Design review of the part built by this model. Coordinates are the model's own, in mm. Give positions to 0.01 mm unless a question says otherwise; leave off trailing zeros. Write each loop counter-clockwise with the first axis right and the second up, starting at its lowest first coordinate (ties: lowest second). Pieces come first, ordered by that corner, then holes. Notation, with made-up numbers: M -5.5,37 L 8.5,37 A18 ccw 8.5,58 Z; hole C 56,65 d5. An arc over 180 degrees is marked long. Use one line per item in the form item = value. Start each with the question number.
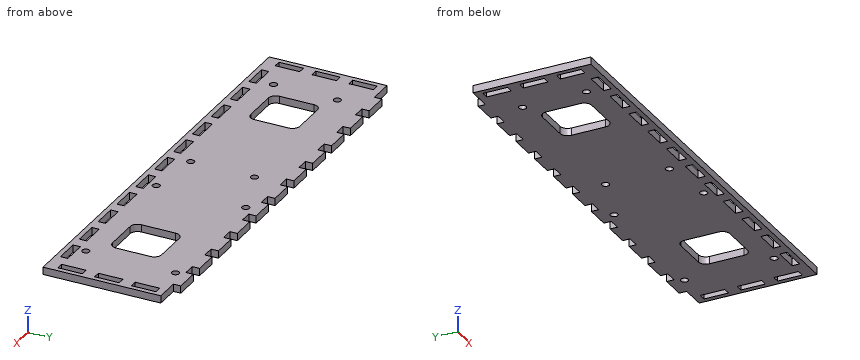
from build123d import *

# Parameters (mm, degrees)
SKETCH_1_W          = 3
SKETCH_1_H          = 10
SKETCH_1_W_2        = 10
SKETCH_1_H_2        = 3
EXTRUDE_1_DEPTH     = 3
SKETCH_2_W          = 20
SKETCH_2_H          = 20
CUT_EXTRUDE_1_DEPTH = 10
FILLET_1_R          = 3
SKETCH_3_R          = 1.5
CUT_EXTRUDE_2_DEPTH = 10


with BuildPart() as part:
    # 草图1 → 凸台-拉伸1 (new body)
    with BuildSketch(Plane.XY):
        Polygon((-90, 24), (-80, 24), (-80, 27), (-70, 27), (-70, 24), (-65, 24), (-65, 27), (-55, 27), (-55, 24), (-50, 24), (-50, 27), (-40, 27), (-40, 24), (-35, 24), (-35, 27), (-25, 27), (-25, 24), (-20, 24), (-20, 27), (-10, 27), (-10, 24), (-5, 24), (-5, 27), (5, 27), (5, 24), (10, 24), (10, 27), (20, 27), (20, 24), (25, 24), (25, 27), (35, 27), (35, 24), (40, 24), (40, 27), (50, 27), (50, 24), (55, 24), (55, 27), (65, 27), (65, 24), (70, 24), (70, 27), (80, 27), (80, 24), (90, 24), (90, -24), (-90, -24), align=None)
        with Locations((-86.5, 1)):
            Rectangle(SKETCH_1_W, SKETCH_1_H, mode=Mode.SUBTRACT)
        with Locations((-86.5, 16)):
            Rectangle(SKETCH_1_W, SKETCH_1_H, mode=Mode.SUBTRACT)
        with Locations((-86.5, -14)):
            Rectangle(SKETCH_1_W, SKETCH_1_H, mode=Mode.SUBTRACT)
        with Locations((86.5, -14)):
            Rectangle(SKETCH_1_W, SKETCH_1_H, mode=Mode.SUBTRACT)
        with Locations((86.5, 1)):
            Rectangle(SKETCH_1_W, SKETCH_1_H, mode=Mode.SUBTRACT)
        with Locations((86.5, 16)):
            Rectangle(SKETCH_1_W, SKETCH_1_H, mode=Mode.SUBTRACT)
        with Locations((-60, -20.5)):
            Rectangle(SKETCH_1_W_2, SKETCH_1_H_2, mode=Mode.SUBTRACT)
        with Locations((-75, -20.5)):
            Rectangle(SKETCH_1_W_2, SKETCH_1_H_2, mode=Mode.SUBTRACT)
        with Locations((-45, -20.5)):
            Rectangle(SKETCH_1_W_2, SKETCH_1_H_2, mode=Mode.SUBTRACT)
        with Locations((-30, -20.5)):
            Rectangle(SKETCH_1_W_2, SKETCH_1_H_2, mode=Mode.SUBTRACT)
        with Locations((-15, -20.5)):
            Rectangle(SKETCH_1_W_2, SKETCH_1_H_2, mode=Mode.SUBTRACT)
        with Locations((0, -20.5)):
            Rectangle(SKETCH_1_W_2, SKETCH_1_H_2, mode=Mode.SUBTRACT)
        with Locations((15, -20.5)):
            Rectangle(SKETCH_1_W_2, SKETCH_1_H_2, mode=Mode.SUBTRACT)
        with Locations((30, -20.5)):
            Rectangle(SKETCH_1_W_2, SKETCH_1_H_2, mode=Mode.SUBTRACT)
        with Locations((45, -20.5)):
            Rectangle(SKETCH_1_W_2, SKETCH_1_H_2, mode=Mode.SUBTRACT)
        with Locations((60, -20.5)):
            Rectangle(SKETCH_1_W_2, SKETCH_1_H_2, mode=Mode.SUBTRACT)
        with Locations((75, -20.5)):
            Rectangle(SKETCH_1_W_2, SKETCH_1_H_2, mode=Mode.SUBTRACT)
    extrude(amount=EXTRUDE_1_DEPTH)

    # 草图2 → 切除-拉伸1 (cut)
    with BuildSketch(Plane.XY.offset(3)):
        with Locations((55, 0)):
            Rectangle(SKETCH_2_W, SKETCH_2_H)
        with Locations((-55, 0)):
            Rectangle(SKETCH_2_W, SKETCH_2_H)
    extrude(amount=-CUT_EXTRUDE_1_DEPTH, mode=Mode.SUBTRACT)

    # 圆角1
    fillet_1_edges = [part.edges().sort_by_distance(p)[0] for p in [
        (65, 10, 1.5),
        (65, -10, 1.5),
        (45, -10, 1.5),
        (45, 10, 1.5),
        (-45, 10, 1.5),
        (-45, -10, 1.5),
        (-65, -10, 1.5),
        (-65, 10, 1.5),
    ]]
    fillet(fillet_1_edges, radius=FILLET_1_R)

    # 草图3 → 切除-拉伸2 (cut)
    with BuildSketch(Plane.XY.offset(3)):
        with Locations((-72, 13)):
            Circle(SKETCH_3_R)
        with Locations((-6, 13)):
            Circle(SKETCH_3_R)
        with Locations((-72, -13)):
            Circle(SKETCH_3_R)
        with Locations((-6, -13)):
            Circle(SKETCH_3_R)
        with Locations((16, 20.75)):
            Circle(SKETCH_3_R)
        with Locations((16, -15.75)):
            Circle(SKETCH_3_R)
        with Locations((72, 20.75)):
            Circle(SKETCH_3_R)
        with Locations((72, -15.75)):
            Circle(SKETCH_3_R)
    extrude(amount=-CUT_EXTRUDE_2_DEPTH, mode=Mode.SUBTRACT)


solid = part.part
1. We need section B-B (y = 8.5). State the section outline as (x, z) points.
2. Clearance check with a flat-ended pin moving along its axis: pin 1 Ø3.5 at (x, y) = (16, -15.75) entering from +Z. State where the tip first meets the part, or that it passes through.
3. To check wall thickness, follow L1, parallel to Y at x = 72, z = 1.4; L2, parallel to X at y = -11, z = 1.95; L3, parallel to X at y = 3.5, z = 1.95. State the ranges of each line that lie inside material, in increasing order.
4. We need section D-D (z = 1.65). Give the number of separate pieces and of enclosed holes in the cut face, and give its area (3 significant figures).
5. We need section A-A (x = 57.5). State the section outline as (y, z) points, and give its area (3 significant figures).
6. We need section C-C (x = -12). State the section outline as (y, z) points, and give its area (3 significant figures).
Answer block:
q1.outline = M -90,0 L -64.6,0 L -64.6,3 L -90,3 Z; M -45.4,0 L 45.4,0 L 45.4,3 L -45.4,3 Z; M 64.6,0 L 90,0 L 90,3 L 64.6,3 Z
q2.pin_1 = 3
q3.L1 = -24 to -22, -19 to -17.25, -14.25 to 19.25, 22.25 to 27
q3.L2 = -90 to -88, -85 to 85, 88 to 90
q3.L3 = -90 to -88, -85 to -65, -45 to 45, 65 to 85, 88 to 90
q4.separate_pieces = 1
q4.enclosed_holes = 27
q4.area = 7,620 mm^2
q5.outline = M -24,0 L -22,0 L -22,3 L -24,3 Z; M -19,0 L -10,0 L -10,3 L -19,3 Z; M 10,0 L 27,0 L 27,3 L 10,3 Z
q5.area = 84.0 mm^2
q6.outline = M -24,0 L -22,0 L -22,3 L -24,3 Z; M -19,0 L 27,0 L 27,3 L -19,3 Z
q6.area = 144 mm^2
